Part model, mm, in its own coordinate system. Round coordinates to 2 decimals unless told otherwise and drop trailing zeros. Write each loop counter-clockwise with the first axis right and the second up, starting at its lowest first coordinate (ties: lowest second). Pieces come first, ordered by that corner, then holes. Notation, with made-up numbers: M -3.75,60 L 3.25,60 A17 ccw 3.25,67 Z; hole C -27,-13.75 d6. An arc over 180 degrees is marked long. One line per question, with ' | ' between items. Start each with the question number.
1) Saw through at D-D (z = 1.35). List the corners of the cut face in (x, y) (3 decimals).
2) Saw through at A-A (y = 0). List the corners of the cut face in (x, z) (3 decimals).
3) Saw through at C-C (x = 1.5). List the corners of the cut face in (y, z) (3 decimals), plus the area to 3 significant figures.
4) Mould opens along Z. For faces 1 (the face through (1, -1.5, 0)), 2 (the face through (4.443, -0.013, 0.282)), 3 (the face through (5.5, 0, 0)), 4 (the face through (0.7, 0, -1.5)) say: pulls with the +Z half, pulls with the -Z half, needs draft (parallel to the pull), parting line crosses it, or undercut.
5) Wall check: probe 1 along Y at (x, z) = (1.5, 0.3) (3 decimals); probe 2 along X at (y, z) = (-0.1, -1); probe 3 along X at (y, z) = (-0.15, -0.3). Give the ranges that are in metal, low to high. Write a range as [from, to].
6) Drop flat-ended pins along their axis: pin 1 Ø1.5 at (x, z) = (4, 0.5) entering from +Y; pin 2 Ø0.9 at (x, z) = (3.5, 0.5) entering from -Y. Give the stop position or say it passes through.
7) Saw through at B-B (z = 0). List the corners of the cut face in (x, y) (3 decimals).
```python
from build123d import *

# Parameters (mm, degrees)
SKETCH1_R                = 0.525
BOSS_EXTRUDE1_DEPTH      = 0.9
BOSS_EXTRUDE2_DEPTH      = 1.5
M1_2X0_25_TAPPED_HOLE1_D = 0.95
CUT_EXTRUDE1_DEPTH       = 7.442049363


with BuildPart() as part:
    # Sketch1 → Boss-Extrude1 (new, symmetric)
    with BuildSketch(Plane(origin=(0, 0, 0), x_dir=(1, 0, 0), z_dir=(0, 1, 0))):
        with BuildLine():
            ThreePointArc((2.64, -1.02), (2.668328157, -1.334164079), (2.4, -1.5))
            Line((2.4, -1.5), (4, -1.5))
            ThreePointArc((4, -1.5), (5.5, 0), (4, 1.5))
            Line((4, 1.5), (2.4, 1.5))
            ThreePointArc((2.4, 1.5), (2.668328157, 1.334164079), (2.64, 1.02))
            ThreePointArc((2.64, 1.02), (2.3, 0), (2.64, -1.02))
        make_face()
        with Locations(Location((4, 0, 0), (0, 0, 270))):
            Circle(SKETCH1_R, mode=Mode.SUBTRACT)
    extrude(amount=BOSS_EXTRUDE1_DEPTH, both=True)

    # Sketch1_4 → Boss-Extrude2 (add, symmetric)
    with BuildSketch(Plane(origin=(0, 0, 0), x_dir=(1, 0, 0), z_dir=(0, 1, 0))):
        with BuildLine():
            Line((-4, 1.5), (-4, -1.5))
            Line((-4, -1.5), (2.4, -1.5))
            ThreePointArc((2.4, -1.5), (2.668328157, -1.334164079), (2.64, -1.02))
            ThreePointArc((2.64, -1.02), (2.3, 0), (2.64, 1.02))
            ThreePointArc((2.64, 1.02), (2.668328157, 1.334164079), (2.4, 1.5))
            Line((2.4, 1.5), (-4, 1.5))
        make_face()
    extrude(amount=BOSS_EXTRUDE2_DEPTH, both=True)

    # M1.2x0.25 Tapped Hole1 (through all)
    with Locations(Plane(origin=(0, 0, -1.5), x_dir=(-1, 0, 0), z_dir=(0, 0, -1))):
        with Locations((-1.5, 0), (1.2, 0)):
            Hole(M1_2X0_25_TAPPED_HOLE1_D / 2)

    # Sketch5 → Cut-Extrude1 (cut, through all)
    with BuildSketch(Plane(origin=(0, 0, -1.5), x_dir=(-1, 0, 0), z_dir=(0, 0, -1))):
        with BuildLine():
            Line((1.2, 1.5), (4, 1.5))
            Line((4, 1.5), (4, -1.5))
            Line((4, -1.5), (1.2, -1.5))
            ThreePointArc((1.2, -1.5), (2.7, 0), (1.2, 1.5))
        make_face()
    extrude(amount=-CUT_EXTRUDE1_DEPTH, mode=Mode.SUBTRACT)


solid = part.part
```
Answer key:
1) outline: M -1.2,-1.5 L 2.66,-1.5 L 2.66,-0.9 L 4.654,-0.9 L 4.654,0.9 L 2.66,0.9 L 2.66,1.5 L -1.2,1.5 A1.5 ccw Z; hole C -1.2,0 d0.95; hole C 1.5,0 d0.95
2) outline: M -2.7,-1.5 L -1.675,-1.5 L -1.675,1.5 L -2.7,1.5 Z; M -0.725,-1.5 L 1.025,-1.5 L 1.025,1.5 L -0.725,1.5 Z; M 1.975,-1.5 L 4,-1.5 A1.5 ccw 4,1.5 L 1.975,1.5 Z; hole C 4,0 d1.05
3) outline: M -1.5,-1.5 L -0.475,-1.5 L -0.475,1.5 L -1.5,1.5 Z; M 0.475,-1.5 L 1.5,-1.5 L 1.5,1.5 L 0.475,1.5 Z | area: 6.15 mm2
4) face 1: needs draft | face 2: undercut | face 3: parting line crosses it | face 4: pulls with the -Z half
5) probe 1: y = [-1.5, -0.475], [0.475, 1.5] | probe 2: x = [-2.7, -1.66], [-0.74, 1.04], [1.96, 5.12] | probe 3: x = [-2.69, -1.65], [-0.75, 1.05], [1.95, 3.57], [4.43, 5.47]
6) pin 1: stops at y = 0.9 | pin 2: stops at y = -0.9
7) outline: M -1.2,-1.5 L 2.3,-1.5 L 2.3,-0.9 L 3.475,-0.9 L 3.475,0.9 L 2.3,0.9 L 2.3,1.5 L -1.2,1.5 A1.5 ccw Z; M 4.525,-0.9 L 5.5,-0.9 L 5.5,0.9 L 4.525,0.9 Z; hole C -1.2,0 d0.95; hole C 1.5,0 d0.95
